Geometry: final body of the model. Coordinates: model frame, mm. A direction names the side the tool comes from. Give positions to 0.01 mm unless a question says otherwise; leave off trailing zeros. Order: outer loops, then holes, each group sorted by start corner. A loop starts at its lowest first (then second) coordinate and runs counter-clockwise, first axis right, second up. Notation, with made-up numbers: (58, -6) -> (63, -6) arc R18 cw to (63, 23) -> close; hole circle Ø7 at (68, -10.75). An arc over 180 degrees is marked (long way). One line per question, with ' | ' between items. Start each with the question number.
(1) Section B-B (y = 0). Return loops of the section in (x, z), then the cut area to 3 significant figures.
(2) Set-up query: faces 1 (the face through (-12, 0, 19.8)), 2 (the face through (-12, 0, 16.1)), 3 (the face through (11.35, 0, 21)), 4 (the face through (11.35, 0, 8)). Return all of +Z, -Z, +X, -X, +Y, -Y with unobstructed straight access to the full face (end or side cutting, diameter ignored); none if empty.
(3) Mould query, pull axis X, two halves, no side actions, for faces 5 (the face through (-6, 0, 30.6)), 6 (the face through (-15.35, 0.07, 17.98)), 7 (the face through (15.9, 0, 18)), 8 (the face through (12.35, 0.07, 17.98)). Classes: +X half, -X half, draft (parallel to the pull), parting line (faces both ways), or undercut.
(4) Section A-A (x = 13.85). Return loops of the section in (y, z).
(5) Section D-D (x = -5.6). Return loops of the section in (y, z).
(6) First-contact query: pin 1 Ø5 at (x, y) = (-13.5, 1.5) entering from +Z; pin 2 Ø3.5 at (x, y) = (14, -1) entering from +Z; pin 3 Ø2 at (y, z) = (-3.5, 13) entering from -X; pin 4 Ø6 at (x, y) = (11.5, 1) entering from -Z. Flat tips, straight axial feed; report the tip coordinate or a pass-through.
(7) Section C-C (y = 3.75). Return loops of the section in (x, z).
(8) Ray query, L1, parallel to Y at x = -13.85, z = 17.7; L2, parallel to Z at x = -13, y = 2; L3, parallel to X at y = -0.5, z = 18. Return the intervals inside material, ascending.
```python
from build123d import *

# Parameters (mm, degrees)
SKETCH1_W           = 22.7
SKETCH1_H           = 12.5
BOSS_EXTRUDE1_DEPTH = 22.8
SKETCH2_W           = 4.55
SKETCH2_H           = 12.5
BOSS_EXTRUDE2_DEPTH = 6.7
SKETCH3_W           = 4.55
SKETCH3_H           = 3
CUT_EXTRUDE1_DEPTH  = 13.5
SKETCH4_R           = 1.5
CUT_EXTRUDE2_DEPTH  = 16.1
SKETCH6_W           = 10.618713929
SKETCH6_H           = 12.5
BOSS_EXTRUDE4_DEPTH = 3.9
SKETCH8_R           = 2.077581334
BOSS_EXTRUDE5_DEPTH = 3.9


with BuildPart() as part:
    # Sketch1 → Boss-Extrude1 (new body)
    with BuildSketch(Plane.XY):
        Rectangle(SKETCH1_W, SKETCH1_H)
    extrude(amount=BOSS_EXTRUDE1_DEPTH)

    # Sketch2 → Boss-Extrude2 (add)
    with BuildSketch(Plane.XY.offset(22.8)):
        with Locations((-13.625, 0)):
            Rectangle(SKETCH2_W, SKETCH2_H)
        with Locations((13.625, 0)):
            Rectangle(SKETCH2_W, SKETCH2_H)
    extrude(amount=-BOSS_EXTRUDE2_DEPTH)

    # Sketch3 → Cut-Extrude1 (cut, through all)
    with BuildSketch(Plane.XZ.offset(6.25)):
        with Locations((-13.625, 21.3)):
            Rectangle(SKETCH3_W, SKETCH3_H)
        with Locations((13.625, 21.3)):
            Rectangle(SKETCH3_W, SKETCH3_H)
    extrude(amount=-CUT_EXTRUDE1_DEPTH, mode=Mode.SUBTRACT)

    # Sketch4 → Cut-Extrude2 (cut)
    with BuildSketch(Plane.XY.offset(19.8)):
        with Locations((13.85, 0)):
            Circle(SKETCH4_R)
        with Locations((-13.85, 0)):
            Circle(SKETCH4_R)
    extrude(amount=-CUT_EXTRUDE2_DEPTH, mode=Mode.SUBTRACT)

    # Sketch6 → Boss-Extrude4 (add)
    with BuildSketch(Plane.XY.offset(22.8)):
        with Locations((-6.040643036, 0)):
            Rectangle(SKETCH6_W, SKETCH6_H)
    extrude(amount=BOSS_EXTRUDE4_DEPTH)

    # Sketch8 → Boss-Extrude5 (add)
    with BuildSketch(Plane.XY.offset(26.7)):
        with Locations((-5.6, 0)):
            Circle(SKETCH8_R)
    extrude(amount=BOSS_EXTRUDE5_DEPTH)


solid = part.part
```
Response:
1) outline: (-15.9, 16.1) -> (-15.35, 16.1) -> (-15.35, 19.8) -> (-15.9, 19.8) -> close; (-12.35, 16.1) -> (-11.35, 16.1) -> (-11.35, 0) -> (11.35, 0) -> (11.35, 16.1) -> (12.35, 16.1) -> (12.35, 19.8) -> (11.35, 19.8) -> (11.35, 22.8) -> (-0.73, 22.8) -> (-0.73, 26.7) -> (-3.52, 26.7) -> (-3.52, 30.6) -> (-7.68, 30.6) -> (-7.68, 26.7) -> (-11.35, 26.7) -> (-11.35, 19.8) -> (-12.35, 19.8) -> close; (15.35, 16.1) -> (15.9, 16.1) -> (15.9, 19.8) -> (15.35, 19.8) -> close | area: 587 mm^2
2) face 1: +Z, -X, +Y, -Y | face 2: -Z, -X, +Y, -Y | face 3: +Z, +X, +Y, -Y | face 4: -Z, +X, +Y, -Y
3) face 5: draft | face 6: undercut | face 7: +X half | face 8: undercut
4) outline: (-6.25, 16.1) -> (-1.5, 16.1) -> (-1.5, 19.8) -> (-6.25, 19.8) -> close; (1.5, 16.1) -> (6.25, 16.1) -> (6.25, 19.8) -> (1.5, 19.8) -> close
5) outline: (-6.25, 0) -> (6.25, 0) -> (6.25, 26.7) -> (2.08, 26.7) -> (2.08, 30.6) -> (-2.08, 30.6) -> (-2.08, 26.7) -> (-6.25, 26.7) -> close
6) pin 1: stops at z = 26.7 | pin 2: stops at z = 19.8 | pin 3: stops at x = -11.35 | pin 4: stops at z = 0
7) outline: (-15.9, 16.1) -> (-11.35, 16.1) -> (-11.35, 0) -> (11.35, 0) -> (11.35, 16.1) -> (15.9, 16.1) -> (15.9, 19.8) -> (11.35, 19.8) -> (11.35, 22.8) -> (-0.73, 22.8) -> (-0.73, 26.7) -> (-11.35, 26.7) -> (-11.35, 19.8) -> (-15.9, 19.8) -> close
8) L1: y = -6.25 to -1.5, 1.5 to 6.25 | L2: z = 16.1 to 19.8 | L3: x = -15.9 to -15.26, -12.44 to 12.44, 15.26 to 15.9
